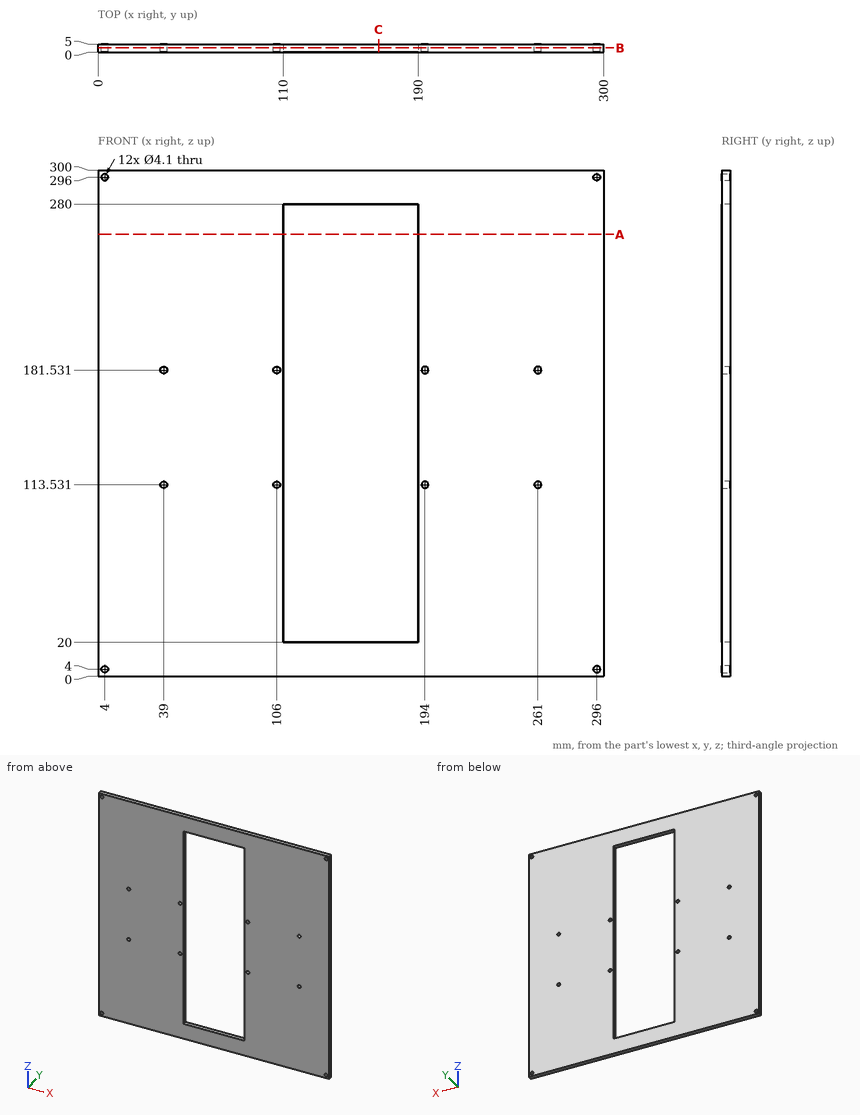
The drawing under review shows one solid part. Ordinate dimensions are in mm from its lowest x, y, z. Coordinates: 2 decimals unless noted, no trailing zeros. Order: outer loops, then holes, each group sorted by start corner. A loop starts at its lowest first (then second) coordinate and runs counter-clockwise, first axis right, second up. Notation, with made-up numbers: M 51.25,-10 L 82.25,-10 A32 ccw 82.25,26 Z; hole C 65.25,36.5 d3. An arc over 180 degrees is marked long. One line per question, with ' | ' between items.
(1) Add section C-C, the plane x = 166.5. Write out the cut boundary in (y, z).
Geometry results:
outline: M 0,0 L 5,0 L 5,20 L 0,20 Z; M 0,280 L 5,280 L 5,300 L 0,300 Z
(2) Add section B-B, the plane y = 2.75. State how many separate pieces and enclosed holes the cut face has, then the cut area to 3 significant figures.
Geometry results:
separate pieces: 1 | enclosed holes: 13 | area: 69,000 mm²
(3) For probe 1 along X at (y, z) = (1, 296); probe 2 along Z at (x, y) = (261, 2.9), list the stretches that pass through material, from the lowest coordinate up. Write a range as from..to.
Geometry results:
probe 1: x = 0..1.95, 6.05..293.95, 298.05..300 | probe 2: z = 0..111.48, 115.58..179.48, 183.58..300
(4) Add section A-A, the plane z = 262. Write out the cut boundary in (x, y).
Geometry results:
outline: M 0,0 L 110,0 L 110,5 L 0,5 Z; M 190,0 L 300,0 L 300,5 L 190,5 Z
